Build history of the part. All positions in model axes, mm. Face numbers are marked on the shaded views. Coordinates: 2 decimals unless noted, no trailing zeros. Order: outer loops, then holes, each group sorted by start corner. A loop starts at its lowest first (then second) coordinate and runs counter-clockwise, first axis right, second up. Notation, with made-up numbers: M 31.25,6 L 88.25,6 A6 cw 88.25,16 Z; hole C 32,-32.5 d4. An arc over 180 degrees is marked long. Write item = value, one per line. Start each with the question number.
Q1. Band-saw the part on B-B on x = -10.75. Write the cut outline in (y, z), plus the area to 3 significant figures.
Q2. Pull direction Y, two halves, no side cores. Call the marked faces 1 and 2: released by +Y, released by -Y, zero draft, split by the parting line, or undercut.
Q3. Band-saw the part on C-C on y = 4.5. Write the cut outline in (x, z).
Q4. Band-saw the part on A-A on x = 2.25. Write the cut outline in (y, z), plus the area to 4 significant figures.
Q5. Pin check, flat tips, straight feed: P1, Ø0.6, axis at y = 6, z = 2, coming from the -X side; P2, Ø7.5, axis at x = 11.5, y = -2.5, coming from the +Z side; P3, Ø1, axis at x = -0.5, y = -4, coming from the +Z side. Stop position of each tip, or through.
Q6. Drill centre lines: probe 1 along Y at (x, z) = (5, 1.95); probe 2 along X at (y, z) = (-1.5, 2.1); probe 3 along X at (y, z) = (-3.25, 1.9). Where is each one in solid material? Low to high.
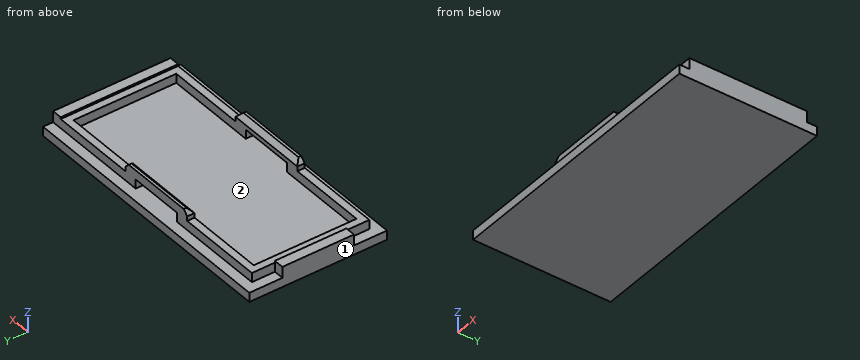
```python
from build123d import *

# Parameters (mm, degrees)
SKETCH_W        = 30
SKETCH_H        = 15
PAD_DEPTH       = 1
SKETCH001_W     = 27.8
SKETCH001_H     = 12.8
SKETCH001_W_2   = 26.2
SKETCH001_H_2   = 11.2
PAD001_DEPTH    = 1
SKETCH002_W     = 1.1
SKETCH002_H     = 7.8
SKETCH002_H_2   = 12.8
PAD002_DEPTH    = 1.2
SKETCH003_W     = 9
SKETCH003_H     = 0.8
PAD003_DEPTH    = 1
SKETCH004_W     = 6
SKETCH004_H     = 1
POCKET_DEPTH    = 13.901
CHAMFER_SIZE    = 0.5
CHAMFER001_SIZE = 0.5


with BuildPart() as part:
    # Sketch → Pad (new body)
    with BuildSketch(Plane.XY):
        Rectangle(SKETCH_W, SKETCH_H)
    extrude(amount=PAD_DEPTH)

    # Sketch001 (on Face6 of Pad) → Pad001 (join)
    with BuildSketch(Plane.XY.offset(1)):
        Rectangle(SKETCH001_W, SKETCH001_H)
        Rectangle(SKETCH001_W_2, SKETCH001_H_2, mode=Mode.SUBTRACT)
    extrude(amount=PAD001_DEPTH)

    # Sketch002 (on Face5 of Pad001) → Pad002 (join)
    with BuildSketch(Plane.XY.offset(1)):
        with Locations((-14.45, 0)):
            Rectangle(SKETCH002_W, SKETCH002_H)
        with Locations((14.45, 0)):
            Rectangle(SKETCH002_W, SKETCH002_H_2)
    extrude(amount=PAD002_DEPTH)

    # Sketch003 (on Face21 of Pad002) → Pad003 (join)
    with BuildSketch(Plane.XY.offset(2)):
        with Locations((0, 6)):
            Rectangle(SKETCH003_W, SKETCH003_H)
        with Locations((0, -6)):
            Rectangle(SKETCH003_W, SKETCH003_H)
    extrude(amount=PAD003_DEPTH)

    # Sketch004 (on Face12 of Pad003) → Pocket (cut, through all)
    with BuildSketch(Plane(origin=(0, 6.4, 0), x_dir=(-1, 0, 0), z_dir=(0, 1, 0))):
        with Locations((0, 1.5)):
            Rectangle(SKETCH004_W, SKETCH004_H)
    extrude(amount=-POCKET_DEPTH, mode=Mode.SUBTRACT)

    # Chamfer
    chamfer_edges = [part.edges().sort_by_distance(p)[0] for p in [
        (-4.5, -6, 3),
        (-4.5, 6, 3),
        (4.5, 6, 3),
        (4.5, -6, 3),
    ]]
    chamfer(chamfer_edges, length=CHAMFER_SIZE)

    # Chamfer001
    chamfer001_edges = [part.edges().sort_by_distance(p)[0] for p in [
        (0, 5.6, 3),
        (0, -5.6, 3),
    ]]
    chamfer(chamfer001_edges, length=CHAMFER001_SIZE)


solid = part.part
```
Recorded:
q1.outline = M -7.5,0 L 7.5,0 L 7.5,1 L 6.4,1 L 6.4,2 L 5.6,2 L 5.6,1 L -5.6,1 L -5.6,2 L -6.4,2 L -6.4,1 L -7.5,1 Z
q1.area = 16.6 mm2
q2.face_1 = zero draft
q2.face_2 = undercut
q3.outline = M -15,0 L 15,0 L 15,2.2 L 13.9,2.2 L 13.9,2 L 13.1,2 L 13.1,1 L -13.1,1 L -13.1,2 L -13.9,2 L -13.9,1 L -15,1 Z
q4.outline = M -7.5,0 L 7.5,0 L 7.5,1 L -7.5,1 Z; M -6.4,2 L -5.6,2 L -5.6,2.5 L -6.1,3 L -6.4,3 Z; M 5.6,2 L 6.4,2 L 6.4,3 L 6.1,3 L 5.6,2.5 Z
q4.area = 16.35 mm2
q5.P1 = -13.9
q5.P2 = 2.2
q5.P3 = 1
q6.probe_1 = -6.4 to -5.6, 5.6 to 6.4
q6.probe_2 = -15 to -13.9, 13.9 to 15
q6.probe_3 = -15 to -13.1, 13.1 to 15
